Work out the finished part from the listing and answer in its coordinate system (mm). Coordinates: 2 decimals unless noted, no trailing zeros. Write each loop counter-clockwise with the first axis right and the second up, starting at its lowest first coordinate (ties: lowest second). Pieces come first, ordered by that corner, then holes. Notation, with made-up numbers: (71, 3) - (123, 3) arc R26 ccw to (123, 23) - close; hole circle Ø8 at (2.25, -31). An arc over 180 degrees is marked (long way). Use a Markdown table: item, result. Add a question column.
(1) The part is cut by section A-A, the plane x = 0. State how many separate pieces and enclosed holes the cut face has, then the cut area to 3 significant figures.
(2) Given pin 1 Ø1.8 at (y, z) = (0, 18.26) entering from -X, flat-ended and moving along its own axis, determine where the tip first touches the part or whether it passes through.
(3) Find the intervals of material crossed by line 1 (Y direction, x = 0.05, z = 24.5); line 2 (Z direction, x = 2.05, y = 1.3); line 3 (Z direction, x = 1.55, y = -0.8), in increasing order. Write a range as from..to.
(4) For a pull along Z with two mould halves and no side action, classify faces 1 (the face through (0, 2.381, 13)), 2 (the face through (0.03, 0.06, 13.38)), 3 (the face through (-0.19, 0.03, 19.97)), 4 (the face through (0, 0, 0)) as released by +Z, released by -Z, zero draft, split by the parting line, or undercut.
(5) The part is cut by section C-C, the plane x = 2.05. Give the vertices of the cut face in (y, z).
(6) The part is cut by section D-D, the plane z = 23.75. Give the vertices of the cut face in (x, y), then the cut area to 3 significant figures.
Autodesk Inventor part; units mm, degrees
ref_plane "YZ Plane" through (0, 0, 0) normal (1, 0, 0) x (0, 1, 0)
ref_plane "XZ Plane" through (0, 0, 0) normal (0, 1, 0) x (-1, 0, 0)
ref_plane "XY Plane" through (0, 0, 0) normal (0, 0, 1) x (1, 0, 0)
sketch "Sketch1" plane through (0, 0, 0) normal (0, 0, 1) x (1, 0, 0)
  line L0 (-2.3812, -2.3813) -> (2.3813, -2.3813)
  line L1 (2.3813, -2.3813) -> (2.3812, 2.3812)
  line L2 (2.3812, 2.3812) -> (-2.3813, 2.3812)
  line L3 (-2.3813, 2.3812) -> (-2.3812, -2.3813)
  line L4 (-2.3812, -2.3813) -> (2.3812, 2.3812) construction
  line L5 (2.3813, -2.3813) -> (-2.3813, 2.3812) construction
  point P0 (0, 0)
  dimension "d0" = 4.7625
  dimension "d1" = 4.7625
extrude "Extrusion1" add sketch "Sketch1" along normal blind 26.9875
sketch "Sketch2" plane through (-2.3813, 2.3812, 0) normal (0, 1, 0) x (1, 0, 0)
  line L0 (2.3813, 0) -> (2.3813, -26.9875) construction
  line L1 (4.7625, -26.9875) -> (0, -26.9875)
  circle A0 centre (2.3813, -2.3813) radius 1.4732
  circle A1 centre (2.3813, -8.7313) radius 1.4732
  circle A2 centre (2.3813, -15.0813) radius 1.4732
  circle A3 centre (2.3813, -21.4313) radius 1.4732
  circle A4 centre (2.3813, -26.1938) radius 1.4493 construction
  line L2 (4.7625, 0) -> (0, 0)
  dimension "d4" = 2.9464
  dimension "d7" = 6.35
  dimension "d12" = 4.7625
  dimension "d13" = 2.3813
extrude "Extrusion2" cut sketch "Sketch2" against normal through all
sketch "Sketch3" plane through (2.3813, -2.3813, 0) normal (1, 0, 0) x (0, 0, -1)
  line L0 (0, 2.3813) -> (-26.9875, 2.3813) construction
  line L1 (-26.9875, 0) -> (-26.9875, 4.7625)
  circle A0 centre (-24.6063, 2.3813) radius 1.4732
  circle A1 centre (-18.2563, 2.3813) radius 1.4732
  circle A2 centre (-11.9063, 2.3813) radius 1.4732
  circle A3 centre (-5.5563, 2.3813) radius 1.4732
  dimension "d16" = 2.9464
  dimension "d17" = 2.3813
  dimension "d20" = 6.35
extrude "Extrusion3" cut sketch "Sketch3" against normal through all
chamfer "Chamfer1" distance 0.1 angle 45 4 edges at (-2.3813, 2.3812, 13.4938) (2.3812, 2.3812, 13.4938) (2.3813, -2.3813, 13.4938) (-2.3812, -2.3813, 13.4938)
equation "\"d1\" = d0"
properties part number "Nut Strip" material "Aluminum 6061"
Model answer:
| question | item | result |
|---|---|---|
| 1 | separate pieces | 5 |
| 1 | enclosed holes | 4 |
| 1 | area | 45.1 mm^2 |
| 2 | pin 1 | through |
| 3 | line 1 | -2.38..-1.47, 1.47..2.38 |
| 3 | line 2 | 0..4.86, 6.25..11.21, 12.6..17.56, 18.95..23.91, 25.3..26.99 |
| 3 | line 3 | 0..4.32, 6.79..10.67, 13.14..17.02, 19.49..23.37, 25.84..26.99 |
| 4 | face 1 | zero draft |
| 4 | face 2 | undercut |
| 4 | face 3 | undercut |
| 4 | face 4 | released by -Z |
| 5 | outline | (-2.38, 0) - (2.38, 0) - (2.38, 26.99) - (-2.38, 26.99) - close; hole circle Ø2.95 at (0, 5.56); hole circle Ø2.95 at (0, 11.91); hole circle Ø2.95 at (0, 18.26); hole circle Ø2.95 at (0, 24.61) |
| 6 | outline | (-2.38, -2.28) - (-2.28, -2.38) - (2.28, -2.38) - (2.38, -2.28) - (2.38, -1.2) - (-2.38, -1.2) - close; (-2.38, 1.2) - (2.38, 1.2) - (2.38, 2.28) - (2.28, 2.38) - (-2.28, 2.38) - (-2.38, 2.28) - close |
| 6 | area | 11.2 mm^2 |
